Here's how the part is built. I have some questions about the finished solid (model axes, mm). A direction names the side the tool comes from. Round coordinates to 2 decimals unless told otherwise and drop trailing zeros. Write each loop counter-clockwise with the first axis right and the second up, starting at its lowest first coordinate (ties: lowest second). Pieces come first, ordered by that corner, then holes. Notation, with made-up numbers: (58, 58) -> (97, 58) arc R32 ccw to (97, 94) -> close; hole circle Ø5 at (66, -24). An arc over 180 degrees is marked (long way). Put each result on its own line as item: value. Start each with the question number.
1) We'd pull the mould along Y, two halves only. Please class faces 4 (the flat face through (-53, -31.75, 1)), 5 (the flat face through (-44.5, -29, 1)), 6 (the flat face through (-45, 8.25, 1)): released by +Y, released by -Y, zero draft, split by the parting line, or undercut.
2) I want a section at A-A, the plane x = -50. List the corners of the cut face in (y, z) for me.
3) Will these pins go through, and if not, where does the flat tip stop? P1, Ø0.8, axis at x = -45, z = 1.5, coming from the +Y side; P2, Ø1.5, axis at y = 17, z = 1.5, coming from the +X side; P3, Ø0.5, axis at x = -45, z = 1, coming from the -Y side.
4) Which directions (+Z, -Z, +X, -X, +Y, -Y) give clear straight access to the entire face, cutting with the end or side of a thin tool? Please do faces 1 (the flat face through (-61, 29, 1)), 2 (the flat face through (-60, -19, 1)), 3 (the flat face through (-45, -28.75, 1)).
5) If I drill on line 1 along Y through (x, z) = (-50, 1.4); line 2 along X through (y, z) = (-11, 0.3); line 3 along Y through (x, z) = (-49, 1.25), over which ranges is the centre line in solid material (lowest first)? Write a range as [from, to].
6) I want a section at B-B, the plane z = 2.25. List the corners of the cut face in (x, y) for me.
7) I want a section at D-D, the plane y = 10. List the corners of the cut face in (x, z) for me.
8) I want a section at C-C, the plane y = 0. List the corners of the cut face in (x, z) for me.
from build123d import *

# Parameters (mm, degrees)
SKETCH1_R           = 1.6
BOSS_EXTRUDE1_DEPTH = 3
FILLET1_R           = 2


with BuildPart() as part:
    # Sketch1 → Boss-Extrude1 (new body)
    with BuildSketch(Plane.XY):
        Polygon((-45.5, 28.75), (-45.5, 8.25), (-44.5, 8.25), (-44.5, -8.25), (-45.5, -8.25), (-45.5, -28.75), (-44.5, -28.75), (-44.5, -31.75), (-61, -31.75), (-61, -28.75), (-60, -28.75), (-60, -8.25), (-61, -8.25), (-61, 8.25), (-60, 8.25), (-60, 28.75), (-61, 28.75), (-61, 31.75), (-44.5, 31.75), (-44.5, 28.75), align=None)
        with Locations((-50, 0)):
            Circle(SKETCH1_R, mode=Mode.SUBTRACT)
    extrude(amount=BOSS_EXTRUDE1_DEPTH)

    # Fillet1
    fillet1_edges = [part.edges().sort_by_distance(p)[0] for p in [
        (-44.5, -31.75, 1.5),
        (-61, -31.75, 1.5),
        (-61, 31.75, 1.5),
        (-44.5, 31.75, 1.5),
    ]]
    fillet(fillet1_edges, radius=FILLET1_R)


solid = part.part
Findings:
1. face 4: released by -Y
1. face 5: zero draft
1. face 6: undercut
2. outline: (-31.75, 0) -> (-1.6, 0) -> (-1.6, 3) -> (-31.75, 3) -> close; (1.6, 0) -> (31.75, 0) -> (31.75, 3) -> (1.6, 3) -> close
3. P1: stops at y = 31.42
3. P2: stops at x = -45.5
3. P3: stops at y = -31.31
4. face 1: +Z, -Z, -X, +Y, -Y
4. face 2: +Z, -Z, -X
4. face 3: +Z, -Z, +X
5. line 1: y = [-31.75, -1.6], [1.6, 31.75]
5. line 2: x = [-60, -45.5]
5. line 3: y = [-31.75, -1.25], [1.25, 31.75]
6. outline: (-61, -29.75) arc R2 ccw to (-59, -31.75) -> (-46.5, -31.75) arc R2 ccw to (-44.5, -29.75) -> (-44.5, -28.75) -> (-45.5, -28.75) -> (-45.5, -8.25) -> (-44.5, -8.25) -> (-44.5, 8.25) -> (-45.5, 8.25) -> (-45.5, 28.75) -> (-44.5, 28.75) -> (-44.5, 29.75) arc R2 ccw to (-46.5, 31.75) -> (-59, 31.75) arc R2 ccw to (-61, 29.75) -> (-61, 28.75) -> (-60, 28.75) -> (-60, 8.25) -> (-61, 8.25) -> (-61, -8.25) -> (-60, -8.25) -> (-60, -28.75) -> (-61, -28.75) -> close; hole circle Ø3.2 at (-50, 0)
7. outline: (-60, 0) -> (-45.5, 0) -> (-45.5, 3) -> (-60, 3) -> close
8. outline: (-61, 0) -> (-51.6, 0) -> (-51.6, 3) -> (-61, 3) -> close; (-48.4, 0) -> (-44.5, 0) -> (-44.5, 3) -> (-48.4, 3) -> close
